Work out the finished part from the listing and answer in its coordinate system (mm). Round coordinates to 2 decimals unless told otherwise and drop trailing zeros. Write each loop counter-clockwise with the first axis right and the second up, starting at its lowest first coordinate (ties: lowest second). Pieces come first, ordered by that corner, then holes. Notation, with made-up numbers: (55.25, -10) -> (80.25, -10) arc R3 ccw to (80.25, -5) -> close; hole circle Ø3 at (-29, 73). An arc over 180 degrees is marked (long way). Answer as a JSON object with one key per item and string values. Group by question number.
from build123d import *

# Parameters (mm, degrees)
EXTRUDE_1_DEPTH     = 1.5
SKETCH_3_R          = 22
EXTRUDE_2_DEPTH     = 1.5
SKETCH_4_R          = 35.070526428
CUT_EXTRUDE_1_DEPTH = 1.5
SKETCH_5_R          = 0.7
CUT_EXTRUDE_2_DEPTH = 1.5
SKETCH_6_R          = 2.5
CUT_EXTRUDE_3_DEPTH = 1.5


with BuildPart() as part:
    # 草图2 → 凸台-拉伸1 (new body)
    with BuildSketch(Plane.XY):
        with BuildLine():
            Line((-6, -20.3), (6, -20.3))
            Line((6, -20.3), (7.479773249, -16.152182272))
            ThreePointArc((7.479773249, -16.152182272), (0, 17.8), (-7.479773249, -16.152182272))
            Line((-7.479773249, -16.152182272), (-6, -20.3))
        make_face()
    extrude(amount=EXTRUDE_1_DEPTH)

    # 草图3 → 凸台-拉伸2 (add)
    with BuildSketch(Plane.XY.offset(1.5)):
        Circle(SKETCH_3_R)
    extrude(amount=EXTRUDE_2_DEPTH)

    # 草图4 → 切除-拉伸1 (cut)
    with BuildSketch(Plane(origin=(0, 0, 0), x_dir=(-1, 0, 0), z_dir=(0, 0, -1))):
        Circle(SKETCH_4_R)
    extrude(amount=-CUT_EXTRUDE_1_DEPTH, mode=Mode.SUBTRACT)

    # 草图5 → 切除-拉伸2 (cut)
    with BuildSketch(Plane(origin=(0, 0, 1.5), x_dir=(-1, 0, 0), z_dir=(0, 0, -1))):
        with Locations((20.5, 0)):
            Circle(SKETCH_5_R)
        with Locations((-10.25, -17.753520778)):
            Circle(SKETCH_5_R)
        with Locations((-10.25, 17.753520778)):
            Circle(SKETCH_5_R)
    extrude(amount=-CUT_EXTRUDE_2_DEPTH, mode=Mode.SUBTRACT)

    # 草图6 → 切除-拉伸3 (cut)
    with BuildSketch(Plane(origin=(0, 0, 1.5), x_dir=(-1, 0, 0), z_dir=(0, 0, -1))):
        Circle(SKETCH_6_R)
    extrude(amount=-CUT_EXTRUDE_3_DEPTH, mode=Mode.SUBTRACT)


solid = part.part
1) A cutting plane is placed at C-C on z = 1.9. Determine the outline of the cut face in (x, y), plus the area to 3 significant figures.
2) A cutting plane is placed at B-B on y = 0. Determine the outline of the cut face in (x, z).
3) For a pull along Y with two mould halves and no side action, classify faces 1 (the face through (-4.769, -21.477, 2.24)), 2 (the face through (0, -5, 1.5)), 3 (the face through (-21.168, 0.21, 2.24)) as released by +Y, released by -Y, zero draft, split by the parting line, or undercut.
4) A cutting plane is placed at D-D on x = 10.25. Determine the outline of the cut face in (y, z).
5) Straight lines are drawn through the part: L1, parallel to Y at x = 0, z = 2.2; L2, parallel to X at y = -1.5, z = 2.25; L3, parallel to X at y = -15.5, z = 2.45. For each, find the intervals that lie inside material, in ascending order.
6) This flat-tipped pin is pushed along its axis until it touches: P1, Ø1.3, axis at x = 10.25, y = 17.75, coming from the -Z side. Where does it stop, or does it pass through?
7) A cutting plane is placed at A-A on x = 0. Determine the outline of the cut face in (y, z), plus the area to 3 significant figures.
Established:
{
 "1": {"outline": "circle Ø44 at (0, 0); hole circle Ø1.4 at (-20.5, 0); hole circle Ø5 at (0, 0); hole circle Ø1.4 at (10.25, -17.75); hole circle Ø1.4 at (10.25, 17.75)", "area": "1,500 mm²"},
 "2": {"outline": "(-22, 1.5) -> (-21.2, 1.5) -> (-21.2, 3) -> (-22, 3) -> close; (-19.8, 1.5) -> (-2.5, 1.5) -> (-2.5, 3) -> (-19.8, 3) -> close; (2.5, 1.5) -> (22, 1.5) -> (22, 3) -> (2.5, 3) -> close"},
 "3": {"face 1": "split by the parting line", "face 2": "zero draft", "face 3": "undercut"},
 "4": {"outline": "(-19.47, 1.5) -> (-18.45, 1.5) -> (-18.45, 3) -> (-19.47, 3) -> close; (-17.05, 1.5) -> (17.05, 1.5) -> (17.05, 3) -> (-17.05, 3) -> close; (18.45, 1.5) -> (19.47, 1.5) -> (19.47, 3) -> (18.45, 3) -> close"},
 "5": {"L1": "y = -22 to -2.5, 2.5 to 22", "L2": "x = -21.95 to -2, 2 to 21.95", "L3": "x = -15.61 to 15.61"},
 "6": {"P1": "passes through"},
 "7": {"outline": "(-22, 1.5) -> (-2.5, 1.5) -> (-2.5, 3) -> (-22, 3) -> close; (2.5, 1.5) -> (22, 1.5) -> (22, 3) -> (2.5, 3) -> close", "area": "58.5 mm²"}
}
